from build123d import *

# Parameters (mm, degrees)
SKETCH2_W                  = 228.6
SKETCH2_H                  = 165.1
BOSS_EXTRUDE1_DEPTH        = 4.7625
F_1_2_0_5_DIAMETER_HOLE1_D = 25.4
SKETCH7_R                  = 66.675
CUT_EXTRUDE4_DEPTH         = 169.123203057
FILLET1_R                  = 6.35
CUT_EXTRUDE5_DEPTH         = 169.123203057
FILLET2_R                  = 4.7625
SKETCH9_R                  = 2.5527
CUT_EXTRUDE6_DEPTH         = 169.123203057
SKETCH10_OUTSIDE_W         = 285.248
SKETCH10_OUTSIDE_H         = 206.251
SKETCH10_OUTSIDE_R         = 63.5
CUT_EXTRUDE7_DEPTH         = 169.123203057
FILLET3_R                  = 6.35
SKETCH11_R                 = 2.5527
CUT_EXTRUDE8_DEPTH         = 133.640575761
CIRPATTERN1_COUNT          = 4


with BuildPart() as part:
    # Sketch2 → Boss-Extrude1 (new body)
    with BuildSketch(Plane.XY):
        with Locations((0, 40.65)):
            Rectangle(SKETCH2_W, SKETCH2_H)
    extrude(amount=BOSS_EXTRUDE1_DEPTH)

    # 1_2 _0.5_ Diameter Hole1 (through all)
    with Locations(Plane.XY.offset(4.7625)):
        with Locations((-38.227, 85.227), (38.227, 85.227), (11.2268, 45.984)):
            Hole(F_1_2_0_5_DIAMETER_HOLE1_D / 2)

    # Sketch7 → Cut-Extrude4 (cut, through all)
    with BuildSketch(Plane(origin=(0, 0, 0), x_dir=(-1, 0, 0), z_dir=(0, 0, -1))):
        with Locations((0, 180.35)):
            Circle(SKETCH7_R)
    extrude(amount=-CUT_EXTRUDE4_DEPTH, mode=Mode.SUBTRACT)

    # Fillet1
    fillet1_edges = [part.edges().sort_by_distance(p)[0] for p in [
        (-114.3, 123.2, 2.38125),
        (114.3, 123.2, 2.38125),
        (114.3, -41.9, 2.38125),
        (-114.3, -41.9, 2.38125),
    ]]
    fillet(fillet1_edges, radius=FILLET1_R)

    # Sketch8 → Cut-Extrude5 (cut, through all)
    with BuildSketch(Plane.XY.offset(4.7625)):
        with BuildLine():
            Line((-107.95, -41.9), (107.95, -41.9))
            ThreePointArc((107.95, -41.9), (112.440128061, -40.040128061), (114.3, -35.55))
            Line((114.3, -35.55), (114.3, -10.15))
            Line((114.3, -10.15), (56.945117879, -10.15))
            ThreePointArc((56.945117879, -10.15), (32.110421547, -23.329546563), (4.1275, -26.053274001))
            Line((4.1275, -26.053274001), (4.1275, 23.1875))
            Line((4.1275, 23.1875), (-53.975, 23.1875))
            Line((-53.975, 23.1875), (-53.975, -10.15))
            Line((-53.975, -10.15), (-114.3, -10.15))
            Line((-114.3, -10.15), (-114.3, -35.55))
            ThreePointArc((-114.3, -35.55), (-112.440128061, -40.040128061), (-107.95, -41.9))
        make_face()
    extrude(amount=-CUT_EXTRUDE5_DEPTH, mode=Mode.SUBTRACT)

    # Fillet2
    fillet2_edges = [part.edges().sort_by_distance(p)[0] for p in [
        (-53.975, 23.1875, 2.38125),
        (4.1275, 23.1875, 2.38125),
        (4.1275, -26.053274001, 2.38125),
        (56.945117879, -10.15, 2.38125),
        (114.3, -10.15, 2.38125),
        (-114.3, -10.15, 2.38125),
        (-53.975, -10.15, 2.38125),
    ]]
    fillet(fillet2_edges, radius=FILLET2_R)

    # Sketch9 → Cut-Extrude6 (cut, through all)
    with BuildSketch(Plane.XY.offset(4.7625)):
        with Locations((-107.95, 116.85)):
            Circle(SKETCH9_R)
        with Locations((-109.5375, -5.3875)):
            Circle(SKETCH9_R)
        with Locations((109.5375, -5.3875)):
            Circle(SKETCH9_R)
        with Locations((107.95, 116.85)):
            Circle(SKETCH9_R)
    extrude(amount=-CUT_EXTRUDE6_DEPTH, mode=Mode.SUBTRACT)

    # Sketch10 outside → Cut-Extrude7 (cut, through all)
    with BuildSketch(Plane.XY.offset(4.7625)):
        with Locations((0, 48.3985)):
            Rectangle(SKETCH10_OUTSIDE_W, SKETCH10_OUTSIDE_H)
        with Locations((11.2268, 45.984)):
            Circle(SKETCH10_OUTSIDE_R, mode=Mode.SUBTRACT)
    extrude(amount=-CUT_EXTRUDE7_DEPTH, mode=Mode.SUBTRACT)

    # Fillet3
    fillet3_edges = [part.edges().sort_by_distance(p)[0] for p in [
        (4.1275, -17.117901235, 2.38125),
        (-29.641139389, 94.585044537, 2.38125),
        (-45.389292566, 74.73931364, 2.38125),
        (-48.040135029, 23.1875, 2.38125),
    ]]
    fillet(fillet3_edges, radius=FILLET3_R)

    # Sketch11 → Cut-Extrude8 (cut, through all)
    with BuildSketch(Plane.XY.offset(4.7625)):
        with Locations((11.2395, 103.136517476)):
            Circle(SKETCH11_R)
    cut_extrude8 = extrude(amount=-CUT_EXTRUDE8_DEPTH, mode=Mode.SUBTRACT)

    # CirPattern1: Cut-Extrude8 ×4 about axis
    cirpattern1_axis = Axis((11.2268, 45.984, 0), (0, 0, 1))
    for i in range(1, CIRPATTERN1_COUNT):
        add(cut_extrude8.rotate(cirpattern1_axis, i * 360 / CIRPATTERN1_COUNT), mode=Mode.SUBTRACT)


solid = part.part
Verification items for the finished model (mm, model axes). A direction names the side the tool comes from. Give positions to 0.01 mm unless a question says otherwise; leave off trailing zeros. Write each loop counter-clockwise with the first axis right and the second up, starting at its lowest first coordinate (ties: lowest second). Pieces come first, ordered by that corner, then holes. Notation, with made-up numbers: M 54.25,-3 L 73.25,-3 A11 ccw 73.25,11 Z; hole C 38.5,82.25 d8. An arc over 180 degrees is marked long. Put each result on its own line as item: value. Start each with the question number.
1. Set-up check for faces 1 (the face through (-47.651, 44.115, 2.415)), 2 (the face through (-22, 23.188, 2)): record each of +Z, -Z, +X, -X, +Y, -Y from which the full face is reachable in a straight line by a thin tool's end or side.
2. Section check C-C (z = 3.65). Give the number of separate pieces and of enclosed holes in the cut face, and give its area (3 significant figures).
3. Section check B-B (x = 12). Record the cut outline in (y, z).
4. Go/stop test with flat-tipped pins: pin 1 Ø1.5 at (y, z) = (86, 3) entering from +X; pin 2 Ø2.5 at (x, z) = (-20.5, 2.5) entering from -Y; pin 3 Ø2 at (x, z) = (-39, 2.5) entering from +Y. Record where each tip stops, or that it passes through.
5. Scan lines: line 1 along X through (y, z) = (50, 3.65); line 2 along X through (y, z) = (37.5, 2.8); line 3 along Y through (x, z) = (-47, 2.35). Record each from-to range of solid material in increasing order. Write a range as [from, to].
6. Section check D-D (x = -34.5). Record the cut outline in (y, z).
7. Section check A-A (y = 40). Record the cut outline in (x, z), and give its area (3 significant figures).
8. Draft check along Y on faces 3 (the face through (4.399, 56.693, 2.348)), 4 (the face through (24.4, 46.9, 4.762)), 5 (the face through (6.007, -15.671, 2.415)). Enter one of: +Y half, -Y half, draft (parallel to the pull), parting line (faces both ways), or undercut.
Answer list:
1. face 1: +Z, -Z
1. face 2: +Z, -Z, -X, -Y
2. separate pieces: 1
2. enclosed holes: 6
2. area: 9,840 mm2
3. outline: M -17.51,0 L -13.6,0 L -13.6,4.76 L -17.51,4.76 Z; M -8.74,0 L 33.31,0 L 33.31,4.76 L -8.74,4.76 Z; M 58.66,0 L 100.7,0 L 100.7,4.76 L 58.66,4.76 Z; M 105.57,0 L 109.48,0 L 109.48,4.76 L 105.57,4.76 Z
4. pin 1: x = 61.13
4. pin 2: y = 23.19
4. pin 3: y = 72.65
5. line 1: [-52.15, -0.82], [23.28, 74.6]
5. line 2: [-51.7, 1.78], [20.68, 74.16]
5. line 3: [24.24, 43.68], [48.31, 70.59]
6. outline: M 23.19,0 L 73.09,0 L 73.09,4.76 L 23.19,4.76 Z
7. outline: M -51.99,0 L 0.02,0 L 0.02,4.76 L -51.99,4.76 Z; M 22.43,0 L 74.44,0 L 74.44,4.76 L 22.43,4.76 Z
7. area: 495 mm2
8. face 3: undercut
8. face 4: draft
8. face 5: -Y half
